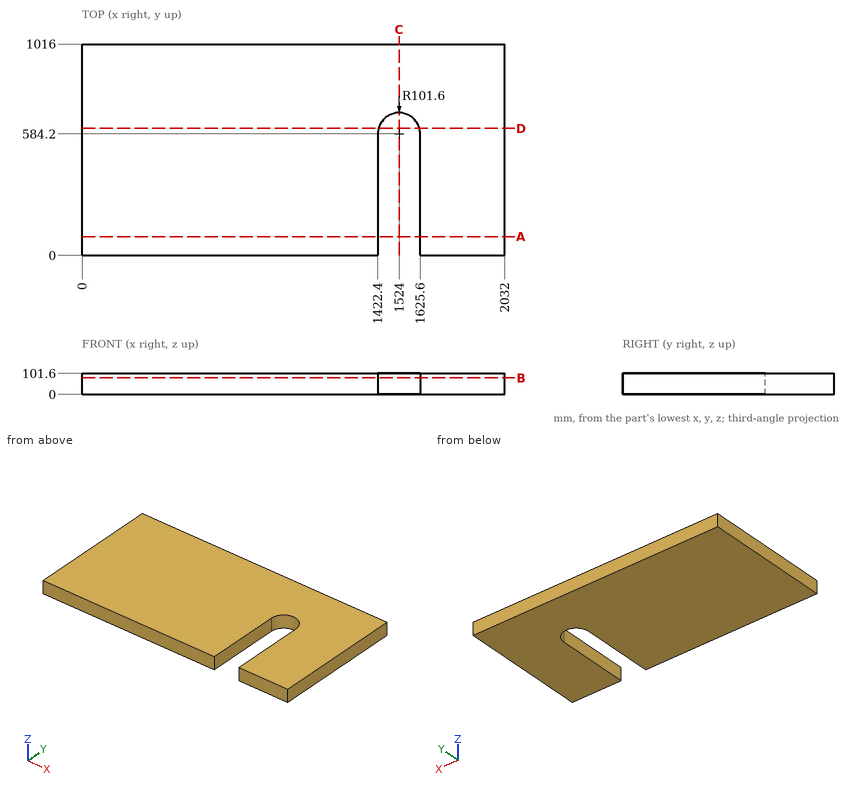
For this review, use the dimensioned drawing (mm, ordinates from the lowest corner) and the shaded views. Give positions to 0.01 mm unless a question says otherwise; leave off trailing zeros. Write each loop counter-clockwise with the first axis right and the second up, starting at its lowest first coordinate (ties: lowest second). Pieces come first, ordered by that corner, then holes. Notation, with made-up numbers: M 12,-11.5 L 32,-11.5 A29 ccw 32,16.5 Z; hole C 56.25,-15.75 d11. An arc over 180 degrees is marked long. Write item = value, one per line. Start each with the question number.
Q1. We need section D-D (y = 610.5). State the section outline as (x, z) points.
Q2. We need section B-B (z = 80). State the section outline as (x, y) points, plus the area to 3 significant figures.
Q3. Clearance check with a flat-ended pin moving along its axis: pin 1 (5 mm diameter, centred on x = 992, y = 206.5, fed in from -Z). State where the tip first meets the part, or that it passes through.
Q4. We need section C-C (x = 1524). State the section outline as (y, z) points.
Q5. We need section A-A (y = 90.5). State the section outline as (x, z) points, plus the area to 3 significant figures.
Q6. For line 1 (X direction, y = 377.5, z = 97); line 2 (Y direction, x = 1542.5, z = 13); line 3 (X direction, y = 669, z = 43.5), list the stretches that pass through material, from the lowest coordinate up.
Result set:
q1.outline = M 0,0 L 1425.86,0 L 1425.86,101.6 L 0,101.6 Z; M 1622.14,0 L 2032,0 L 2032,101.6 L 1622.14,101.6 Z
q2.outline = M 0,0 L 1422.4,0 L 1422.4,584.2 A101.6 cw 1625.6,584.2 L 1625.6,0 L 2032,0 L 2032,1016 L 0,1016 Z
q2.area = 1,930,000 mm2
q3.pin_1 = 0
q4.outline = M 685.8,0 L 1016,0 L 1016,101.6 L 685.8,101.6 Z
q5.outline = M 0,0 L 1422.4,0 L 1422.4,101.6 L 0,101.6 Z; M 1625.6,0 L 2032,0 L 2032,101.6 L 1625.6,101.6 Z
q5.area = 186,000 mm2
q6.line_1 = 0 to 1422.4, 1625.6 to 2032
q6.line_2 = 684.1 to 1016
q6.line_3 = 0 to 1468.04, 1579.96 to 2032
